Check sheet for the drawn part. Datum: minimum x, y, z corner. Units: mm. A direction names the side the tool comes from. Give positions to 0.01 mm unless a question says otherwise; leave off trailing zeros. Order: outer loops, then holes, each group sorted by start corner. A loop starts at its lowest first (then second) coordinate and runs counter-clockwise, first axis right, second up. Notation, with made-up numbers: (70, -29.75) - (125, -29.75) arc R25 cw to (125, 2.25) - close; hole circle Ø10 at (36, 3.25). An arc over 180 degrees is marked (long way). Answer as a JSON object with one key per item and string values. Group by question number.
(1) Thickness scan on line 1 (Z direction, x = 8.5, y = 24); line 2 (X direction, y = 24.5, z = 13.75); line 3 (Z direction, x = 7, y = 18.25). Record the ranges inside material, lowest first.
(2) Section check C-C (z = 18). Record the boundary of the cut face in (x, y).
(3) Section check A-A (y = 21.5). Record the boundary of the cut face in (x, z).
(4) Access from +Z, -Z, +X, -X, +Y, -Y to the whole of each face (thin tool, end or side, straight path). Record for the marked faces 1 and 2.
(5) Section check B-B (x = 8). Record the boundary of the cut face in (y, z), then the cut area to 3 significant figures.
(6) Depth check by flat-ended pin: pin 1 Ø4 at (y, z) = (15, 22) entering from -X; pin 2 Ø4 at (x, y) = (12, 11) entering from +Z; pin 3 Ø7 at (y, z) = (9.5, 14.5) entering from -X. Enter the tip coordinate at first touch or a pass-through.
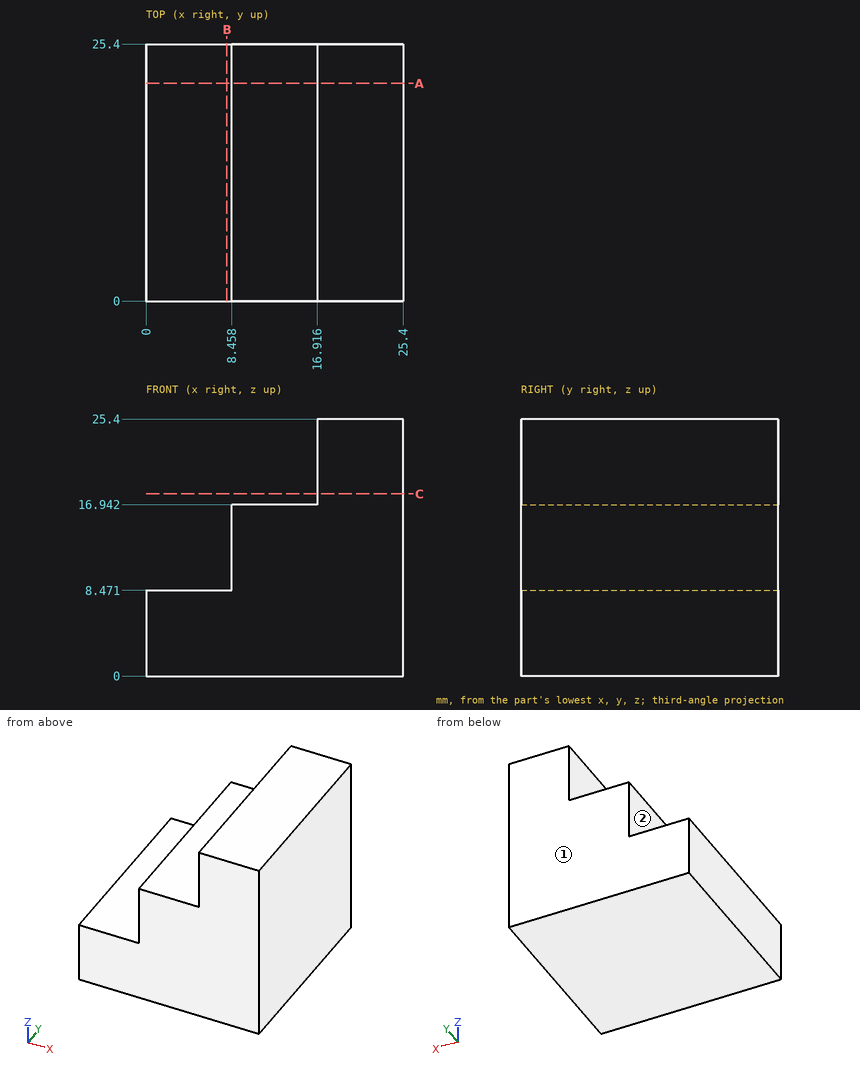
Solutions:
{
 "1": {"line 1": "z = 0 to 16.94", "line 2": "x = 8.46 to 25.4", "line 3": "z = 0 to 8.47"},
 "2": {"outline": "(16.92, 0) - (25.4, 0) - (25.4, 25.4) - (16.92, 25.4) - close"},
 "3": {"outline": "(0, 0) - (25.4, 0) - (25.4, 25.4) - (16.92, 25.4) - (16.92, 16.94) - (8.46, 16.94) - (8.46, 8.47) - (0, 8.47) - close"},
 "4": {"face 1": "+Z, -Z, +X, -X, +Y", "face 2": "+Z, -X, +Y, -Y"},
 "5": {"outline": "(0, 0) - (25.4, 0) - (25.4, 8.47) - (0, 8.47) - close", "area": "215 mm2"},
 "6": {"pin 1": "stops at x = 16.92", "pin 2": "stops at z = 16.94", "pin 3": "stops at x = 8.46"}
}
